```python
from build123d import *

# Parameters (mm, degrees)
F1_DEPTH = 50
F3_DEPTH = 100
F5_DEPTH = 100
F6_R     = 2.5
F7_DEPTH = 6
F8_R     = 5
F9_SIZE  = 0.99999


# Not quite as in the source:
# - a fillet or chamfer is up to 0.001 mm smaller than in the source, because OpenCascade refuses the exact size


with BuildPart() as f1:
    # F0 (on Right) → F1 (new body, symmetric)
    with BuildSketch(Plane.YZ):
        Polygon((0, 7), (0, 0), (-60, 0), (-60, -6), (-11.5, -6), (-11.5, -74), (5, -74), (5, -71), (0, -71), (0, -72), (-5.5, -72), (-5.5, -5), (4.5, -5), (4.5, 7), align=None)
    extrude(amount=F1_DEPTH, both=True)

    # F2 (on face) → F3 (cut, through all)
    with BuildSketch(Plane.YZ.offset(50)):
        Polygon((4.5, 7), (2.25, 7), (4.5, 0), align=None)
    extrude(amount=-F3_DEPTH, mode=Mode.SUBTRACT)

    # F4 (on face) → F5 (cut, through all)
    with BuildSketch(Plane.YZ.offset(50)):
        Polygon((0, -71), (0, -72), (2.5, -71), align=None)
        Polygon((5, -71), (2.5, -71), (5, -72.108708322), align=None)
    extrude(amount=-F5_DEPTH, mode=Mode.SUBTRACT)

    # F6 (on face) → F7 (cut, through all)
    with BuildSketch(Plane.XY):
        with Locations((-30, -35)):
            Circle(F6_R)
        with Locations((30, -35)):
            Circle(F6_R)
    extrude(amount=-F7_DEPTH, mode=Mode.SUBTRACT)

    # F8
    f8_edges = [f1.edges().sort_by_distance(p)[0] for p in [
        (0, -11.5, -6),
    ]]
    fillet(f8_edges, radius=F8_R)

    # F9 (size 1 in the source; OpenCascade refuses exactly that, so slightly less here)
    f9_edges = [f1.edges().sort_by_distance(p)[0] for p in [
        (50, -11.5, -42.5),
        (50, -12.964466, -7.464466),
        (50, -3.25, -74),
        (50, -38.25, -6),
        (50, 5, -73.054354),
        (50, -60, -3),
        (50, 3.75, -71.554354),
        (50, -30, 0),
        (50, 1.25, -71.5),
        (50, 0, 3.5),
        (50, -2.75, -72),
        (50, 1.125, 7),
        (50, -5.5, -38.5),
        (50, 3.375, 3.5),
        (50, -0.5, -5),
        (50, 4.5, -2.5),
        (-50, -11.5, -42.5),
        (-50, -12.964466, -7.464466),
        (-50, -3.25, -74),
        (-50, -38.25, -6),
        (-50, 5, -73.054354),
        (-50, -60, -3),
        (-50, 3.75, -71.554354),
        (-50, -30, 0),
        (-50, 1.25, -71.5),
        (-50, 0, 3.5),
        (-50, -2.75, -72),
        (-50, 1.125, 7),
        (-50, -5.5, -38.5),
        (-50, 3.375, 3.5),
        (-50, -0.5, -5),
        (-50, 4.5, -2.5),
    ]]
    chamfer(f9_edges, length=F9_SIZE)


solid = f1.part
```
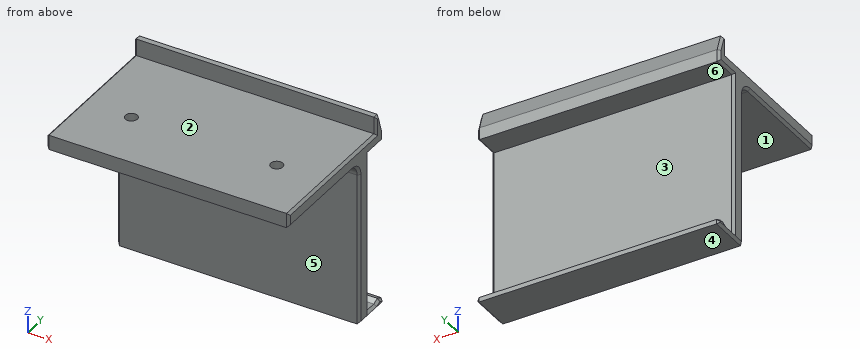
Source: CAD feature listing. Evaluate the final solid. Frame: model axes, mm. Face numbers are marked on the shaded views. A direction names the side the tool comes from. Round coordinates to 2 decimals unless told otherwise and drop trailing zeros. Order: outer loops, then holes, each group sorted by start corner. A loop starts at its lowest first (then second) coordinate and runs counter-clockwise, first axis right, second up. Notation, with made-up numbers: (12.5, 16) -> (49.5, 16) arc R9 cw to (49.5, 20) -> close; hole circle Ø3 at (89, 8). An arc over 180 degrees is marked (long way). One line per item, written item: value. Start each with the question number.
Q1. Section query B-B (y = -35). Return the cut outline in (x, z).
Q2. Draft query along Z for the marked faces 1, 2 and 3. Return one class per face: pulls with the +Z half, pulls with the -Z half, needs draft (parallel to the pull), parting line crosses it, or undercut.
Q3. Section query C-C (z = -66). Return the cut outline in (x, y).
Q4. Pin query (flat end, axial travel): pin 1 (4.5 mm diameter, centred on x = -2, y = -3.5, fed in from +Z); pin 2 (5.5 mm diameter, centred on x = -4.5, z = 3.5, fed in from -Y); pin 3 (5.5 mm diameter, centred on x = 1.5, z = -1.5, fed in from +Y); pin 4 (4.5 mm diameter, centred on x = 30, y = -35, fed in from -Z). Return the tip coordinate at first contact, or that it passes through.
Q5. Section query D-D (x = 8). Return the cut outline in (y, z), plus the area to 3 significant figures.
Q6. Material intervals for probe 1 along Z at (x, y) = (-45, -1); probe 2 along Z at (x, y) = (9.5, -29); probe 3 along Y at (x, z) = (22, -45.5), sorted ascending.
Q7. Access query for the marked faces 4, 5 and 6. Directions: +Z, -Z, +X, -X, +Y, -Y. A direction counts if a zero-diameter tool reaches every point of the face in a straight line with its end or side. Return the directions, or none.
Q8. Section query A-A (x = -30). Return the cut outline in (y, z).
Findings below:
1. outline: (-50, -5) -> (-49, -6) -> (-32.5, -6) -> (-32.5, 0) -> (-49, 0) -> (-50, -1) -> close; (-27.5, -6) -> (27.5, -6) -> (27.5, 0) -> (-27.5, 0) -> close; (32.5, -6) -> (49, -6) -> (50, -5) -> (50, -1) -> (49, 0) -> (32.5, 0) -> close
2. face 1: pulls with the -Z half
2. face 2: pulls with the +Z half
2. face 3: undercut
3. outline: (-50, -10.5) -> (-49, -11.5) -> (49, -11.5) -> (50, -10.5) -> (50, -6.5) -> (49, -5.5) -> (-49, -5.5) -> (-50, -6.5) -> close
4. pin 1: z = 0
4. pin 2: y = 0
4. pin 3: y = 4.5
4. pin 4: through
5. outline: (-60, -6) -> (-16.5, -6) arc R5 cw to (-11.5, -11) -> (-11.5, -74) -> (5, -74) -> (5, -72.11) -> (2.5, -71) -> (0, -72) -> (-5.5, -72) -> (-5.5, -5) -> (4.5, -5) -> (4.5, 0) -> (2.25, 7) -> (0, 7) -> (0, 0) -> (-60, 0) -> close
5. area: 837 mm²
6. probe 1: -74 to -72, -5 to 0
6. probe 2: -6 to 0
6. probe 3: -11.5 to -5.5
7. face 4: -Z, +X, -X, +Y, -Y
7. face 5: -Z, +X, -X, -Y
7. face 6: +X, -X, +Y
8. outline: (-60, -6) -> (-37.5, -6) -> (-37.5, 0) -> (-60, 0) -> close; (-32.5, -6) -> (-16.5, -6) arc R5 cw to (-11.5, -11) -> (-11.5, -74) -> (5, -74) -> (5, -72.11) -> (2.5, -71) -> (0, -72) -> (-5.5, -72) -> (-5.5, -5) -> (4.5, -5) -> (4.5, 0) -> (2.25, 7) -> (0, 7) -> (0, 0) -> (-32.5, 0) -> close
